Here's how the part is built. I have some questions about the finished solid (model axes, mm). Round coordinates to 2 decimals unless told otherwise and drop trailing zeros. Loops run counter-clockwise (first coordinate to the right, second up) from the corner with the lowest first, then second, coordinate; pieces in that order, holes last. Notation, with made-up numbers: M 86,26 L 118,26 A9 ccw 118,32 Z; hole C 66,-19.75 d9. An arc over 180 degrees is marked long. Use a Markdown table: item, result.
from build123d import *

# Parameters (mm, degrees)
SKETCH1_R           = 0.4
SKETCH1_R_2         = 2
BOSS_EXTRUDE1_DEPTH = 1.5


with BuildPart() as part:
    # Sketch1 → Boss-Extrude1 (new body)
    with BuildSketch(Plane(origin=(0, 0, 0), x_dir=(1, 0, 0), z_dir=(0, 1, 0))):
        Polygon((-28, -26.5), (28, -26.5), (28, 26.5), (28, 36.5), (-38, 36.5), (-38, -26.5), align=None)
        with Locations((-23.2, 24.2)):
            Circle(SKETCH1_R, mode=Mode.SUBTRACT)
        with Locations((-20.7, 24.2)):
            Circle(SKETCH1_R, mode=Mode.SUBTRACT)
        with Locations((-18.2, 24.2)):
            Circle(SKETCH1_R, mode=Mode.SUBTRACT)
        with Locations((-15.7, 24.2)):
            Circle(SKETCH1_R, mode=Mode.SUBTRACT)
        with Locations((-13.2, 24.2)):
            Circle(SKETCH1_R, mode=Mode.SUBTRACT)
        with Locations((-10.7, 24.2)):
            Circle(SKETCH1_R, mode=Mode.SUBTRACT)
        with Locations((-8.2, 24.2)):
            Circle(SKETCH1_R, mode=Mode.SUBTRACT)
        with Locations((-5.7, 24.2)):
            Circle(SKETCH1_R, mode=Mode.SUBTRACT)
        with Locations((-10.7, -24.2)):
            Circle(SKETCH1_R, mode=Mode.SUBTRACT)
        with Locations((-13.2, -24.2)):
            Circle(SKETCH1_R, mode=Mode.SUBTRACT)
        with Locations((-15.7, -24.2)):
            Circle(SKETCH1_R, mode=Mode.SUBTRACT)
        with Locations((-18.2, -24.2)):
            Circle(SKETCH1_R, mode=Mode.SUBTRACT)
        with Locations((-20.7, -24.2)):
            Circle(SKETCH1_R, mode=Mode.SUBTRACT)
        with Locations((-23.2, -24.2)):
            Circle(SKETCH1_R, mode=Mode.SUBTRACT)
        with Locations((6.8, -24.2)):
            Circle(SKETCH1_R, mode=Mode.SUBTRACT)
        with Locations((4.3, -24.2)):
            Circle(SKETCH1_R, mode=Mode.SUBTRACT)
        with Locations((1.8, -24.2)):
            Circle(SKETCH1_R, mode=Mode.SUBTRACT)
        with Locations((-0.7, -24.2)):
            Circle(SKETCH1_R, mode=Mode.SUBTRACT)
        with Locations((-3.2, -24.2)):
            Circle(SKETCH1_R, mode=Mode.SUBTRACT)
        with Locations((-5.7, -24.2)):
            Circle(SKETCH1_R, mode=Mode.SUBTRACT)
        with Locations((-0.85, 24.2)):
            Circle(SKETCH1_R, mode=Mode.SUBTRACT)
        with Locations((1.65, 24.2)):
            Circle(SKETCH1_R, mode=Mode.SUBTRACT)
        with Locations((4.15, 24.2)):
            Circle(SKETCH1_R, mode=Mode.SUBTRACT)
        with Locations((6.65, 24.2)):
            Circle(SKETCH1_R, mode=Mode.SUBTRACT)
        with Locations((9.15, 24.2)):
            Circle(SKETCH1_R, mode=Mode.SUBTRACT)
        with Locations((11.65, 24.2)):
            Circle(SKETCH1_R, mode=Mode.SUBTRACT)
        with Locations((14.15, 24.2)):
            Circle(SKETCH1_R, mode=Mode.SUBTRACT)
        with Locations((16.65, 24.2)):
            Circle(SKETCH1_R, mode=Mode.SUBTRACT)
        with Locations((-22, 31.5)):
            Circle(SKETCH1_R_2, mode=Mode.SUBTRACT)
        with Locations((23, 31.5)):
            Circle(SKETCH1_R_2, mode=Mode.SUBTRACT)
        with Locations((-33, -21.5)):
            Circle(SKETCH1_R_2, mode=Mode.SUBTRACT)
    extrude(amount=BOSS_EXTRUDE1_DEPTH)


solid = part.part
1. For pin 1 Ø4 at (x, z) = (-24.5, -11) entering from -Y, with a flat end and sliding along its axis, tell me the tip position at first contact or that it passes through.
Answer sheet:
| item | result |
|---|---|
| pin 1 | y = 0 |
2. Imagine slicing it at A-A, the plane x = -33. Write out the boundary of the cut face in (y, z), then the cut area to 3 significant figures.
Answer sheet:
| item | result |
|---|---|
| outline | M 0,-36.5 L 1.5,-36.5 L 1.5,19.5 L 0,19.5 Z; M 0,23.5 L 1.5,23.5 L 1.5,26.5 L 0,26.5 Z |
| area | 88.5 mm2 |
3. I need wall thicknesses on probe 1 along Z at (x, y) = (-18.2, 0.6); probe 2 along Z at (x, y) = (-20.7, 0.9); probe 3 along Z at (x, y) = (-33, 0.55). Which ranges of each line are inside material? Lowest first, please. Write a range as from..to.
Answer sheet:
| item | result |
|---|---|
| probe 1 | -36.5..-24.6, -23.8..23.8, 24.6..26.5 |
| probe 2 | -36.5..-33.02, -29.98..-24.6, -23.8..23.8, 24.6..26.5 |
| probe 3 | -36.5..19.5, 23.5..26.5 |
4. We'd pull the mould along Z, two halves only. Please class faces 1 (the face through (-5, 1.5, -5)), 2 (the face through (-31.092, 0.74, 20.899)), 3 (the face through (-5, 1, 26.5)), 4 (the face through (22.566, 0.74, -29.548)): +Z half, -Z half, draft (parallel to the pull), parting line (faces both ways), or undercut.
Answer sheet:
| item | result |
|---|---|
| face 1 | draft |
| face 2 | undercut |
| face 3 | +Z half |
| face 4 | undercut |
5. Imagine slicing it at C-C, the plane z = -30.5. Write out the boundary of the cut face in (x, y), then the cut area to 3 significant figures.
Answer sheet:
| item | result |
|---|---|
| outline | M -38,0 L -23.73,0 L -23.73,1.5 L -38,1.5 Z; M -20.27,0 L 21.27,0 L 21.27,1.5 L -20.27,1.5 Z; M 24.73,0 L 28,0 L 28,1.5 L 24.73,1.5 Z |
| area | 88.6 mm2 |
6. Imagine slicing it at B-B, the plane z = 21.5. Write out the boundary of the cut face in (x, y).
Answer sheet:
| item | result |
|---|---|
| outline | M -38,0 L -35,0 L -35,1.5 L -38,1.5 Z; M -31,0 L 28,0 L 28,1.5 L -31,1.5 Z |
